Design review of the part built by this model. Coordinates are the model's own, in mm. Face numbers are marked on the shaded views. A direction names the side the tool comes from. Give positions to 0.01 mm unless a question says otherwise; leave off trailing zeros. Write each loop counter-clockwise with the first axis right and the second up, starting at its lowest first coordinate (ties: lowest second). Pieces come first, ordered by that corner, then holes. Notation, with made-up numbers: (-38.5, 61.5) -> (-14.5, 61.5) arc R10 ccw to (-14.5, 80.5) -> close; hole circle Ø10 at (-28, 14). An arc over 180 degrees is marked (long way). Return JSON: item names as keys, results as strings. Group by question number.
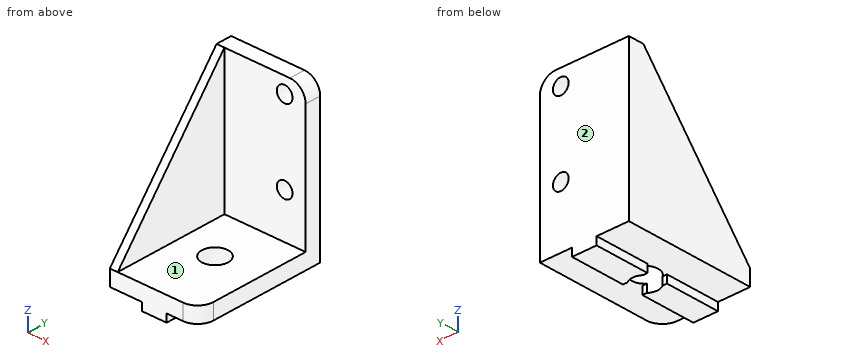
from build123d import *

# Parameters (mm, degrees)
BOSS_EXTRU_1_DEPTH           = 12.5
ENL_V_MAT_EXTRU_1_DEPTH      = 34.966383385
ENL_V_MAT_EXTRU_1_DEPTH_BACK = 34.966383385
ESQUISSE2_R                  = 2.5
ESQUISSE5_W                  = 1.5
ESQUISSE5_H                  = 4
ENL_V_MAT_EXTRU_3_DEPTH      = 35.263282096
ESQUISSE6_W                  = 17
ESQUISSE6_H                  = 30
ESQUISSE6_R                  = 1.5
BOSS_EXTRU_2_DEPTH           = 3
ENL_V_MAT_EXTRU_4_DEPTH      = 37.006943775
CONG_1_R                     = 3


with BuildPart() as part:
    # Esquisse1 → Boss.-Extru.1 (new, symmetric)
    with BuildSketch(Plane(origin=(0, 0, 0), x_dir=(1, 0, 0), z_dir=(0, 1, 0))):
        Polygon((2.35, 0), (8.5, 0), (8.5, -3), (-7, -3), (-7, -30), (-8.5, -30), (-8.5, 0), (-2.35, 0), (-2.35, 1.5), (2.35, 1.5), align=None)
    extrude(amount=BOSS_EXTRU_1_DEPTH, both=True)

    # Esquisse2 → Enlèv. mat.-Extru.1 (cut, two sides: drawn at the far end of the back side and taken through both)
    with BuildSketch(Plane(origin=(-1.372446517, 0, 0), x_dir=(1, 0, 0), z_dir=(0, 0, 1)).offset(-ENL_V_MAT_EXTRU_1_DEPTH_BACK)):
        with Locations(Location((1.372446517, 0, 0), (0, 0, 340.051556411))):
            Circle(ESQUISSE2_R)
    extrude(amount=ENL_V_MAT_EXTRU_1_DEPTH + ENL_V_MAT_EXTRU_1_DEPTH_BACK, mode=Mode.SUBTRACT)

    # Esquisse5 → Enlèv. mat.-Extru.3 (cut, through all)
    with BuildSketch(Plane.ZY.offset(2.35)):
        with Locations((-0.75, 0)):
            Rectangle(ESQUISSE5_W, ESQUISSE5_H)
    extrude(amount=-ENL_V_MAT_EXTRU_3_DEPTH, mode=Mode.SUBTRACT)

    # Esquisse6 → Boss.-Extru.2 (add)
    with BuildSketch(Plane(origin=(0, 12.5, 0), x_dir=(1, 0, 0), z_dir=(0, 1, 0))):
        with Locations((0, -15)):
            Rectangle(ESQUISSE6_W, ESQUISSE6_H)
        with Locations(Location((4.5, -27, 0), (0, 0, 270))):
            Circle(ESQUISSE6_R, mode=Mode.SUBTRACT)
        with Locations(Location((4.5, -11.5, 0), (0, 0, 270))):
            Circle(ESQUISSE6_R, mode=Mode.SUBTRACT)
    extrude(amount=-BOSS_EXTRU_2_DEPTH)

    # Esquisse7 → Enlèv. mat.-Extru.4 (cut, through all)
    with BuildSketch(Plane(origin=(-7, 0, 0), x_dir=(0, 0, -1), z_dir=(1, 0, 0))):
        Polygon((-30, 9.5), (-3, -12.5), (-30, -12.5), align=None)
    extrude(amount=-ENL_V_MAT_EXTRU_4_DEPTH, mode=Mode.SUBTRACT)

    # Congé1
    cong_1_edges = [part.edges().sort_by_distance(p)[0] for p in [
        (8.5, -12.5, 1.5),
        (8.5, 11, 30),
    ]]
    fillet(cong_1_edges, radius=CONG_1_R)


solid = part.part
Q1. Take a section at D-D, the plane x = -5.25. Give the boundary of the cut face in (y, z).
Q2. Take a section at B-B, the plane y = 0.75. Give the boundary of the cut face in (x, z), plus the area to 3 significant figures.
Q3. For L1, parallel to X at y = 11.45, z = 11.5; L2, parallel to Z at x = 2.25, y = 2.25; L3, parallel to Z at x = 4.25, y = 0.5, list the stretches that pass through material, from the lowest coordinate up. Write a range as from..to.
Q4. Insertion check: pin 1 (4 mm diameter, centred on x = 0, y = 0, fed in from -Z); pin 2 (2 mm diameter, centred on x = 4.5, y = 3, fed in from +Z); pin 3 (11 mm diameter, centred on y = -2, z = 20.5, fed in from +X). Each pin has a flat end and moves straight along its axis. Give the tip position at first contact, or say it passes through.
Q5. Take a section at C-C, the plane z = 1. Give the boundary of the cut face in (x, y).
Q6. Tool access review of the marked faces 1 and 2: name each direction out of +Z, -Z, +X, -X, +Y, -Y from which nothing blocks a thin tool from reaching the whole face with its end or side.
Q7. Take a section at A-A, the plane z = 26.5. Give the boundary of the cut face in (x, y), plus the area to 3 significant figures.
Final values:
{
 "1": {"outline": "(-12.5, 0) -> (12.5, 0) -> (12.5, 30) -> (9.5, 30) -> (9.5, 3) -> (-12.5, 3) -> close"},
 "2": {"outline": "(-8.5, 0) -> (-2.38, 0) -> (-2.38, 3) -> (-7, 3) -> (-7, 19.26) -> (-8.5, 19.26) -> close; (2.38, 0) -> (8.5, 0) -> (8.5, 3) -> (2.38, 3) -> close", "area": "61.1 mm²"},
 "3": {"L1": "x = -8.5..3, 6..8.5", "L2": "z = -1.5..3", "L3": "z = 0..3"},
 "4": {"pin 1": "passes through", "pin 2": "stops at z = 3", "pin 3": "stops at x = -7"},
 "5": {"outline": "(-8.5, -12.5) -> (5.5, -12.5) arc R3 ccw to (8.5, -9.5) -> (8.5, 12.5) -> (-8.5, 12.5) -> close; hole circle Ø5 at (0, 0)"},
 "6": {"face 1": "+Z, +X, -Y", "face 2": "+Z, -Z, +X, -X, +Y"},
 "7": {"outline": "(-8.5, 6.65) -> (-7, 6.65) -> (-7, 9.5) -> (3.09, 9.5) -> (3.09, 12.5) -> (-8.5, 12.5) -> close; (5.91, 9.5) -> (8.5, 9.5) -> (8.5, 12.5) -> (5.91, 12.5) -> close", "area": "46.8 mm²"}
}
